Can you work these out from the model? Positions are in its coordinate system, mm. Face numbers are marked on the shaded views. Coordinates: 2 decimals unless noted, no trailing zeros. Order: outer loops, then holes, each group sorted by start corner. A loop starts at its lowest first (then second) coordinate and runs counter-clockwise, first axis right, second up. Notation, with made-up numbers: (-2, -5) -> (12, -5) arc R37 cw to (12, 31) -> close; hole circle Ø8 at (-9, -37.75). An arc over 180 degrees is marked (long way). Return JSON: item names as keys, results as strings. Group by question number.
1) If we section it at A-A, the plane x = 0: Please give me the cut outline in (y, z).
2) For pin 1 (4 mm diameter, centred on x = 11, y = 13.5, fed in from +Z); pin 2 (7 mm diameter, centred on x = 32.3, z = 32.3, fed in from -Y); pin 3 (2 mm diameter, centred on x = -23, z = -21.5, fed in from -Y), each with a flat end and sliding along its axis, tell me the tip position at first contact or that it passes through.
3) Thinking about a two-plate mould opening in X: for the marked faces 1 and 2, which applies, +X half, -X half, draft (parallel to the pull), parting line (faces both ways), or undercut?
4) If we section it at B-B, the plane z = 18: Please give me the cut outline in (x, y), then the cut area to 3 significant figures.
5) If I drill on probe 1 along Y at (x, z) = (17.5, 35); probe 2 along Y at (x, z) = (-34.5, -31.5); probe 3 along Z at (x, y) = (18, 65), over which ranges is the centre line in solid material (lowest first)? Write a range as from..to.
6) If we section it at C-C, the plane y = 34: Please give me the cut outline in (x, z).
7) If we section it at D-D, the plane x = 12.5: Please give me the cut outline in (y, z), then the cut area to 3 significant figures.
from build123d import *

# Parameters (mm, degrees)
SKETCH1_R                 = 40
BOSS_EXTRUDE1_DEPTH       = 70
SKETCH2_W                 = 95
SKETCH2_H                 = 95
BOSS_EXTRUDE2_DEPTH       = 6
SKETCH3_R                 = 40
SKETCH3_R_2               = 38.709273032
CUT_EXTRUDE1_DEPTH        = 1
SKETCH4_R                 = 3
BOSS_EXTRUDE3_DEPTH       = 20
FILLET1_R                 = 8
SKETCH6_R                 = 3.519560707
SKETCH6_R_2               = 3
CUT_EXTRUDE3_DEPTH        = 5
CUT_EXTRUDE4_REACH        = 123.169
CUT_EXTRUDE4_START_RADIUS = 40
CUT_EXTRUDE4_END_RADIUS   = 40
SKETCH8_W                 = 29.147137568
SKETCH8_H                 = 8.22098752
BOSS_EXTRUDE5_DEPTH       = 4
SKETCH10_R                = 2.25
CUT_EXTRUDE5_DEPTH        = 34


with BuildPart() as part:
    # Sketch1 → Boss-Extrude1 (new body)
    with BuildSketch(Plane(origin=(0, 0, 0), x_dir=(1, 0, 0), z_dir=(0, 1, 0))):
        with Locations(Location((0, 0, 0), (0, 0, 270))):
            Circle(SKETCH1_R)
    extrude(amount=BOSS_EXTRUDE1_DEPTH)

    # Sketch2 → Boss-Extrude2 (add)
    with BuildSketch(Plane(origin=(0, 70, 0), x_dir=(1, 0, 0), z_dir=(0, 1, 0))):
        Rectangle(SKETCH2_W, SKETCH2_H)
    extrude(amount=BOSS_EXTRUDE2_DEPTH)

    # Sketch3 → Cut-Extrude1 (cut)
    with BuildSketch(Plane(origin=(0, 76, 0), x_dir=(1, 0, 0), z_dir=(0, 1, 0))):
        with Locations(Location((0, 0, 0), (0, 0, 270))):
            Circle(SKETCH3_R)
        with Locations(Location((0, 0, 0), (0, 0, 270))):
            Circle(SKETCH3_R_2, mode=Mode.SUBTRACT)
    extrude(amount=-CUT_EXTRUDE1_DEPTH, mode=Mode.SUBTRACT)

    # Sketch4 → Boss-Extrude3 (add)
    with BuildSketch(Plane(origin=(0, 76, 0), x_dir=(1, 0, 0), z_dir=(0, 1, 0))):
        with Locations(Location((0, 0, 0), (0, 0, 270))):
            Circle(SKETCH4_R)
    extrude(amount=BOSS_EXTRUDE3_DEPTH)

    # Fillet1
    fillet1_edges = [part.edges().sort_by_distance(p)[0] for p in [
        (47.5, 73, 47.5),
        (47.5, 73, -47.5),
        (-47.5, 73, -47.5),
        (-47.5, 73, 47.5),
    ]]
    fillet(fillet1_edges, radius=FILLET1_R)

    # Sketch6 → Cut-Extrude3 (cut)
    with BuildSketch(Plane(origin=(0, 76, 0), x_dir=(1, 0, 0), z_dir=(0, 1, 0))):
        with Locations(Location((0, 0, 0), (0, 0, 270))):
            Circle(SKETCH6_R)
        with Locations(Location((0, 0, 0), (0, 0, 270))):
            Circle(SKETCH6_R_2, mode=Mode.SUBTRACT)
    extrude(amount=-CUT_EXTRUDE3_DEPTH, mode=Mode.SUBTRACT)

    # Cut-Extrude4: from a cylinder face, 123.169 long prism both ways, kept between that surface and its translate by the depth
    cut_extrude4_start = Plane(origin=(0, 20.055809, 0), z_dir=(0, -1, 0)) * Cylinder(CUT_EXTRUDE4_START_RADIUS, 327.338, mode=Mode.PRIVATE)
    cut_extrude4_end = Plane(origin=(0, 20.055809, -4), z_dir=(0, -1, 0)) * Cylinder(CUT_EXTRUDE4_END_RADIUS, 327.338, mode=Mode.PRIVATE)
    # Sketch8 → Cut-Extrude4 (cut, from a surface)
    with BuildSketch(Plane.XY, mode=Mode.PRIVATE) as cut_extrude4_sk1:
        with Locations((0, 20.055809212)):
            Rectangle(SKETCH8_W, SKETCH8_H)
    cut_extrude4_tool1 = extrude(cut_extrude4_sk1.sketch, amount=CUT_EXTRUDE4_REACH, both=True, mode=Mode.PRIVATE)
    add(((cut_extrude4_tool1 & cut_extrude4_start) - cut_extrude4_end).solids().sort_by_distance((0, 20.055809, 35.250652))[0], mode=Mode.SUBTRACT)

    # Sketch9 → Boss-Extrude5 (add)
    with BuildSketch(Plane.XZ):
        with BuildLine():
            ThreePointArc((-25.622676251, -4.384366141), (-27.880429407, -0.093420807), (-25.772900348, 4.273269294))
            Line((-25.772900348, 4.273269294), (-27.319093183, 6.289872554))
            ThreePointArc((-27.319093183, 6.289872554), (-29.604344551, 3.506882349), (-30.422381519, 0))
            ThreePointArc((-30.422381519, 0), (-29.542433802, -3.629669529), (-27.097976665, -6.453397238))
            Line((-27.097976665, -6.453397238), (-25.622676251, -4.384366141))
        make_face()
    boss_extrude5 = extrude(amount=BOSS_EXTRUDE5_DEPTH)

    # Mirror1: Boss-Extrude5 across plane
    add(boss_extrude5.mirror(Plane(origin=(0, 0, 0), x_dir=(0, 0, 1), z_dir=(1, 0, 0))))

    # Sketch10 → Cut-Extrude5 (cut)
    with BuildSketch(Plane(origin=(0, 76, 0), x_dir=(1, 0, 0), z_dir=(0, 1, 0))):
        with Locations(Location((-32.295599691, 32.295599691, 0), (0, 0, 270))):
            Circle(SKETCH10_R)
        with Locations(Location((32.295599691, 32.295599691, 0), (0, 0, 270))):
            Circle(SKETCH10_R)
        with Locations(Location((32.295599691, -32.295599691, 0), (0, 0, 270))):
            Circle(SKETCH10_R)
        with Locations(Location((-32.295599691, -32.295599691, 0), (0, 0, 270))):
            Circle(SKETCH10_R)
    extrude(amount=-CUT_EXTRUDE5_DEPTH, mode=Mode.SUBTRACT)


solid = part.part
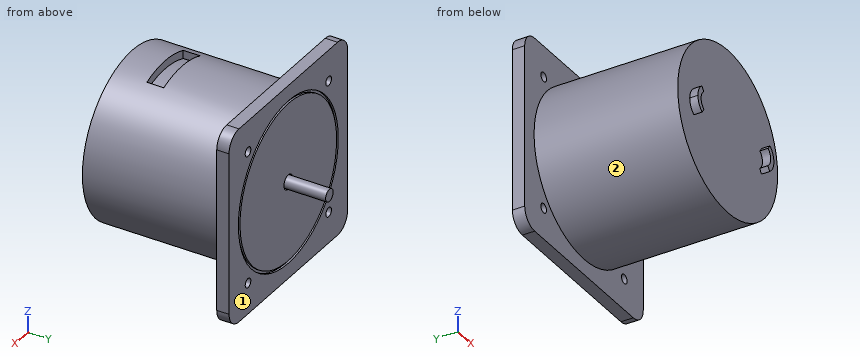
Result sheet:
{
 "1": {"outline": "(0, -40) -> (70, -40) -> (70, -47.5) -> (76, -47.5) -> (76, -40) -> (75, -40) -> (75, -38.71) -> (76, -38.71) -> (76, -3.52) -> (71, -3.52) -> (71, -3) -> (96, -3) -> (96, 3) -> (71, 3) -> (71, 3.52) -> (76, 3.52) -> (76, 38.71) -> (75, 38.71) -> (75, 40) -> (76, 40) -> (76, 47.5) -> (70, 47.5) -> (70, 40) -> (24.17, 40) -> (24.17, 36) -> (15.95, 36) -> (15.95, 40) -> (0, 40) -> close"},
 "2": {"pin 1": "stops at z = 38.97", "pin 2": "stops at y = 70", "pin 3": "stops at y = 0"},
 "3": {"face 1": "draft", "face 2": "parting line"},
 "4": {"outline": "(-47.5, 70) -> (-35.72, 70) -> (-35.72, 0) -> (35.72, 0) -> (35.72, 70) -> (47.5, 70) -> (47.5, 76) -> (35.72, 76) -> (35.72, 75) -> (34.27, 75) -> (34.27, 76) -> (-34.27, 76) -> (-34.27, 75) -> (-35.72, 75) -> (-35.72, 76) -> (-47.5, 76) -> close", "area": "5,570 mm2"},
 "5": {"probe 1": "y = 0..75", "probe 2": "y = 70..76", "probe 3": "z = -35.72..35.72"},
 "6": {"outline": "circle Ø80 at (0, 0)"},
 "7": {"outline": "(0, -38) -> (70, -38) -> (70, -47.5) -> (76, -47.5) -> (76, -38) -> (75, -38) -> (75, -36.64) -> (76, -36.64) -> (76, 36.64) -> (75, 36.64) -> (75, 38) -> (76, 38) -> (76, 47.5) -> (70, 47.5) -> (70, 38) -> (24.17, 38) -> (24.17, 34) -> (15.95, 34) -> (15.95, 38) -> (0, 38) -> close", "area": "5,850 mm2"}
}
